Autodesk Inventor part; units mm, degrees
ref_plane "YZ Plane" through (0, 0, 0) normal (1, 0, 0) x (0, 1, 0)
ref_plane "XZ Plane" through (0, 0, 0) normal (0, 1, 0) x (-1, 0, 0)
ref_plane "XY Plane" through (0, 0, 0) normal (0, 0, 1) x (1, 0, 0)
sketch "Sketch2" plane through (0, 0, 0) normal (0, 1, 0) x (-1, 0, 0)
  arc A0 (762, -479.9355) -> (-762, -479.9355) centre (0, 0) ccw
  line L0 (900.5455, 0) -> (762, 0)
  line L1 (762, -479.9355) -> (-762, -479.9355)
  dimension "d8" = 1524
extrude "Extrusion1" add sketch "Sketch2" along normal blind 63.5
sketch "Sketch4" plane through (0, 63.5, 0) normal (0, 1, 0) x (1, 0, 0)
  arc A0 (-762, 479.9355) -> (762, 479.9355) centre (0, 0) ccw
  line L0 (762, 479.9355) -> (-762, 479.9355)
  arc A1 (-762, 479.9355) -> (762, 479.9355) centre (0, 0) ccw
  line L1 (-762, 479.9355) -> (762, 479.9355)
  line L2 (-790.3185, 352.9355) -> (-828.5038, 352.9355)
  line L3 (-790.3185, 352.9355) -> (-790.3185, 225.9355)
  line L4 (-790.3185, 225.9355) -> (-871.7427, 225.9355)
  dimension "d15" = 127
extrude "Extrusion4" add sketch "Sketch4" along normal blind 381 contours L2 L3 L4 A0
sketch "Sketch5" plane through (0, 63.5, 0) normal (0, 1, 0) x (1, 0, 0)
  line L0 (-790.3185, 225.9355) -> (-871.7427, 225.9355)
  arc A0 (-762, 479.9355) -> (762, 479.9355) centre (0, 0) ccw
  arc A1 (-762, 479.9355) -> (762, 479.9355) centre (0, 0) ccw
  arc A2 (-871.7427, 225.9355) -> (762, 479.9355) centre (0, 0) ccw
  line L1 (-871.7427, 225.9355) -> (-790.3185, 225.9355)
  line L2 (-790.3185, 225.9355) -> (-790.3185, -28.0645)
  line L3 (-790.3185, -28.0645) -> (-900.108, -28.0645)
  line L4 (-790.3185, -28.0645) -> (-790.3185, -155.0645)
  line L5 (-790.3185, -155.0645) -> (-887.0948, -155.0645)
  line L6 (762, 479.9355) -> (-762, 479.9355)
  line L7 (762, 479.9355) -> (-762, 479.9355)
  dimension "d23" = 254
  dimension "d24" = 127
extrude "Extrusion6" add sketch "Sketch5" along normal blind 381 contours L4 L5 A0 L3
sketch "Sketch6" plane through (0, 63.5, 0) normal (0, 1, 0) x (1, 0, 0)
  arc A0 (-762, 479.9355) -> (762, 479.9355) centre (0, 0) ccw
  line L0 (762, 479.9355) -> (-762, 479.9355)
  arc A1 (-762, 479.9355) -> (762, 479.9355) centre (0, 0) ccw
  line L1 (-762, 479.9355) -> (762, 479.9355)
  line L2 (-790.3185, -155.0645) -> (-790.3185, -431.7161)
  arc A2 (-887.0948, -155.0645) -> (762, 479.9355) centre (0, 0) ccw
  line L3 (-790.3185, -431.7161) -> (-688.5633, -355.7235)
  line L4 (-688.5633, -355.7235) -> (-612.5707, -457.4787)
  line L5 (-612.5707, -457.4787) -> (-721.537, -538.8567)
  dimension "d27" = 127
  dimension "d28" = 127
  dimension "d29" = 127
  dimension "d30" = 90
  dimension "d31" = 90
extrude "Extrusion7" add sketch "Sketch6" along normal blind 381 contours L3 L4 L5 A0
sketch "Sketch7" plane through (0, 63.5, 0) normal (0, 1, 0) x (1, 0, 0)
  arc A0 (-762, 479.9355) -> (762, 479.9355) centre (0, 0) ccw
  line L0 (-762, 479.9355) -> (762, 479.9355)
  arc A1 (-721.537, -538.8567) -> (762, 479.9355) centre (0, 0) ccw
  line L1 (-540.1977, -716.7108) -> (-439.217, -613.7513)
  line L2 (-439.217, -613.7513) -> (-348.5473, -702.6783)
  line L3 (-348.5473, -702.6783) -> (-433.5292, -789.3254)
  line L4 (-540.1977, -716.7108) -> (-542.3554, -718.9108)
  arc A2 (-762, 479.9355) -> (762, 479.9355) centre (0, 0) ccw
  dimension "d34" = 254
  dimension "d35" = 127
  dimension "d36" = 90
extrude "Extrusion8" add sketch "Sketch7" along normal blind 381 contours L4 L1 L2 L3 A0
sketch "Sketch8" plane through (0, 63.5, 0) normal (0, 1, 0) x (1, 0, 0)
  arc A0 (-762, 479.9355) -> (762, 479.9355) centre (0, 0) ccw
  line L0 (762, 479.9355) -> (-762, 479.9355)
  line L1 (762, 479.9355) -> (-762, 479.9355)
  arc A1 (-733.4235, 429.1355) -> (733.4235, 429.1355) centre (0, 0) ccw
  line L2 (-733.4235, 429.1355) -> (733.4235, 429.1355)
  dimension "d39" = 50.8
extrude "Extrusion9" cut sketch "Sketch8" along normal blind 381 contours L2 A1
properties part number "Nest-ver2-1111-2021"
Verification items for the finished model (mm, model axes). A direction names the side the tool comes from. Coordinates: 2 decimals unless noted, no trailing zeros. Write each loop counter-clockwise with the first axis right and the second up, starting at its lowest first coordinate (ties: lowest second). Pieces come first, ordered by that corner, then holes. Notation, with made-up numbers: (7.5, 51) - (63.5, 51) arc R9 cw to (63.5, 63) - close; hole circle Ø7 at (70.25, 13.5). An arc over 180 degrees is marked (long way). One line per question, with ' | ' between items. Start each with the question number.
1. Section check A-A (y = 315). Enter the section's corners in (x, z), plus the area to 3 significant figures.
2. Material ranges on line 1 along Y through (x, z) = (-764, -189.5); line 2 along Z through (x, y) = (-423.5, 44); line 3 along X through (y, z) = (146.5, 440), recorded low to high.
3. Section check C-C (z = 51.5). Enter the section's corners in (x, y), plus the area to 3 significant figures.
4. Access from +Z, -Z, +X, -X, +Y, -Y to the whole of each face (thin tool, end or side, straight path). Record for faces 1 (the cylindrical face through (-716.545, 251.333, 456.762)), 2 (the flat face through (-809, 251, -352.936)), 3 (the flat face through (-874, 251, 28.064)), 4 (the flat face through (-700.901, 251.333, 523.445)), 5 (the cylindrical face through (-844.672, 251.333, 92.714)).
5. Gauge pin test, flat ends, axial feed: P1, Ø12, axis at y = 137, z = 710, coming from the +X side; P2, Ø6, axis at x = -33, z = -129, coming from the -Y side; P3, Ø1, axis at x = -595.5, z = 115, coming from the +Y side. Record the tip position at first contact, or that the pin passes through.
6. Section check B-B (x = 0). Enter the section's corners in (y, z), plus the area to 3 significant figures.
7. Draft check along Z on faces 6 (the flat face through (-845, 251, -225.936)), 7 (the cylindrical face through (-452.038, 251.333, 719.534)), 8 (the cylindrical face through (-726.172, 122.435, 532.594)). Enter one of: released by +Z, released by -Z, zero draft, split by the parting line, or undercut.
8. Section check D-D (y = 35). Enter the section's corners in (x, z).
Computed values:
1) outline: (-900.11, 28.06) - (-849.28, 28.06) arc R849.75 cw to (-835.48, 155.06) - (-887.09, 155.06) arc R900.55 ccw to start; (-871.74, -225.94) arc R900.55 ccw to (-828.5, -352.94) - (-790.32, -352.94) - (-790.32, -312.19) arc R849.75 cw to (-819.16, -225.94) - close; (-790.32, 431.72) - (-749.18, 400.99) arc R849.75 cw to (-680.83, 508.46) - (-721.54, 538.86) arc R900.55 ccw to start; (-542.36, 718.91) - (-540.2, 716.71) - (-506.47, 682.32) arc R849.75 cw to (-396.5, 751.57) - (-433.53, 789.33) arc R900.55 ccw to start | area: 26,100 mm²
2) line 1: 0 to 63.5 | line 2: -479.94 to 794.75 | line 3: -785.74 to -726.96
3) outline: (-899.07, 0) - (899.07, 0) - (899.07, 63.5) - (-848.18, 63.5) - (-848.18, 444.5) - (-899.07, 444.5) - close | area: 134,000 mm²
4) face 1: -Z, +X, +Y | face 2: -Z, +X, -X, +Y | face 3: +X, -X, +Y | face 4: +Z, +X, +Y | face 5: +X, +Y
5) P1: x = -457.61 | P2: y = 0 | P3: y = 63.5
6) outline: (0, -479.94) - (63.5, -479.94) - (63.5, 900.55) - (0, 900.55) - close | area: 87,700 mm²
7) face 6: undercut | face 7: released by -Z | face 8: split by the parting line
8) outline: (-762, -479.94) - (762, -479.94) arc R900.55 ccw (long way) to start
